The model under review builds one solid part; all positions refer to its coordinate system, in mm. A direction names the side the tool comes from. Round coordinates to 2 decimals unless told otherwise and drop trailing zeros. Order: outer loops, then holes, each group sorted by start corner. A loop starts at its lowest first (then second) coordinate and runs counter-clockwise, first axis right, second up.
1) Clearance check with flat-ended pins moving along their axes: P1, Ø1.8, axis at y = 20, z = 15.5, coming from the -X side; P2, Ø6.5, axis at y = 16, z = -17, coming from the +X side. State where each tip first meets the part, or that it passes through.
2) To check wall thickness, follow L1, parallel to Z at x = -11.5, y = 15.75; L2, parallel to X at y = 9.5, z = 17; L3, parallel to Y at x = -26.5, z = 7. State the ranges of each line that lie inside material, in increasing order.
3) Consider section D-D (y = 22.25). Give the boundary of the cut face in (x, z).
4) Machinability: for faces 4 (the face through (-9, 15, -17)), 5 (the face through (-22, 15, 17)), 6 (the face through (36, 3, 19)), 7 (the face through (-16, 15, -13)), which of the approach directions +Z, -Z, +X, -X, +Y, -Y give a long, thin tool a straight path to every point of the face, cutting with its end or side? Answer none if there is none.
5) Consider section B-B (z = -3.5). Give the boundary of the cut face in (x, y), then the cut area to 3 significant figures.
6) Consider section C-C (x = -4). Give the boundary of the cut face in (y, z).
7) Mouldability with a two-part tool opening along Z and no side actions: class faces 1 (the face through (-38, 2, 0)), 2 (the face through (-16, 15, 13)), 3 (the face through (-7, 4, 20)) as pulls with the +Z half, pulls with the -Z half, needs draft (parallel to the pull), parting line crosses it, or undercut.
8) Consider section A-A (y = 8). Give the boundary of the cut face in (x, z).
from build123d import *

# Parameters (mm, degrees)
SKETCH_1_W          = 76
SKETCH_1_H          = 40
EXTRUDE_1_DEPTH     = 6
SKETCH_2_W          = 13
SKETCH_2_H          = 40
EXTRUDE_2_DEPTH     = 19
SKETCH_3_W          = 13
SKETCH_3_H          = 26
CUT_EXTRUDE_1_DEPTH = 19
FILLET_1_R          = 4
FILLET_2_R          = 1
FILLET_3_R          = 1
FILLET_4_R          = 5
FILLET_5_R          = 1
FILLET_6_R          = 1
FILLET_7_R          = 0.4


with BuildPart() as part:
    # Эскиз1 → Бобышка-Вытянуть1 (new body)
    with BuildSketch(Plane(origin=(0, 0, 0), x_dir=(1, 0, 0), z_dir=(0, 1, 0))):
        Rectangle(SKETCH_1_W, SKETCH_1_H)
    extrude(amount=EXTRUDE_1_DEPTH)

    # Эскиз2 → Бобышка-Вытянуть2 (add)
    with BuildSketch(Plane(origin=(0, 6, 0), x_dir=(1, 0, 0), z_dir=(0, 1, 0))):
        with Locations((-15.5, 0)):
            Rectangle(SKETCH_2_W, SKETCH_2_H)
    extrude(amount=EXTRUDE_2_DEPTH)

    # Эскиз3 → Вырез-Вытянуть1 (cut)
    with BuildSketch(Plane(origin=(0, 25, 0), x_dir=(1, 0, 0), z_dir=(0, 1, 0))):
        with Locations((-15.5, 0)):
            Rectangle(SKETCH_3_W, SKETCH_3_H)
    extrude(amount=-CUT_EXTRUDE_1_DEPTH, mode=Mode.SUBTRACT)

    # Скругление1
    fillet_1_edges = [part.edges().sort_by_distance(p)[0] for p in [
        (-15.5, 25, 20),
        (-15.5, 25, -20),
    ]]
    fillet(fillet_1_edges, radius=FILLET_1_R)

    # Скругление2
    fillet_2_edges = [part.edges().sort_by_distance(p)[0] for p in [
        (-22, 15.5, -13),
        (-9, 15.5, -13),
        (-15.5, 25, -13),
    ]]
    fillet(fillet_2_edges, radius=FILLET_2_R)

    # Скругление3
    fillet_3_edges = [part.edges().sort_by_distance(p)[0] for p in [
        (-22, 15.5, 13),
        (-9, 15.5, 13),
        (-15.5, 25, 13),
    ]]
    fillet(fillet_3_edges, radius=FILLET_3_R)

    # Скругление4
    fillet_4_edges = [part.edges().sort_by_distance(p)[0] for p in [
        (38, 3, 20),
        (-38, 3, 20),
        (-38, 3, -20),
        (38, 3, -20),
    ]]
    fillet(fillet_4_edges, radius=FILLET_4_R)

    # Скругление5
    fillet_5_edges = [part.edges().sort_by_distance(p)[0] for p in [
        (-38, 6, 0),
        (-27.5, 6, 20),
        (-36.535533906, 6, 18.535533906),
        (-36.535533906, 6, -18.535533906),
        (-27.5, 6, -20),
    ]]
    fillet(fillet_5_edges, radius=FILLET_5_R)

    # Скругление6
    fillet_6_edges = [part.edges().sort_by_distance(p)[0] for p in [
        (12, 6, -20),
        (38, 6, 0),
        (36.535533906, 6, -18.535533906),
        (36.535533906, 6, 18.535533906),
        (12, 6, 20),
    ]]
    fillet(fillet_6_edges, radius=FILLET_6_R)

    # Скругление7
    # the kernel refuses this fillet: 0.4 mm, written as the material it adds along each edge
    with BuildSketch(Plane(origin=(-22, 6, -19), x_dir=(-1, 0, 0), z_dir=(0, 0, 1)), Plane(origin=(-9, 6, 19), x_dir=(1, 0, 0), z_dir=(0, 0, -1)), Plane(origin=(-9, 6, -14), x_dir=(1, 0, 0), z_dir=(0, 0, -1)), Plane(origin=(-22, 6, 14), x_dir=(-1, 0, 0), z_dir=(0, 0, 1))) as fillet_7_piece_1:
        with BuildLine():
            CenterArc((FILLET_7_R, -FILLET_7_R), FILLET_7_R, 90, 90)
            Line((0, -FILLET_7_R), (0, 0))
            Line((0, 0), (FILLET_7_R, 0))
        make_face()
    extrude(amount=5)
    with BuildSketch(Plane(origin=(-22, 5, -19), x_dir=(0, 1, 0), z_dir=(0, 0, 1))) as fillet_7_piece_2_section:
        with BuildLine():
            CenterArc((1 + FILLET_7_R, FILLET_7_R), FILLET_7_R, 180, 90)
            Line((1, FILLET_7_R), (1, 0))
            Line((1, 0), (1 + FILLET_7_R, 0))
        make_face()
    fillet_7_piece_2 = revolve(axis=Axis((-22, 5, -19), (-1, 0, 0)), revolution_arc=147.318795695, mode=Mode.PRIVATE)
    fillet_7_piece_2 = split(fillet_7_piece_2, bisect_by=Plane(origin=(-22.06536945, 6.084454663, -20), z_dir=(0, 0, 1)), keep=Keep.TOP, mode=Mode.PRIVATE)
    add(fillet_7_piece_2)
    with BuildSketch(Plane(origin=(-22, 5, 19), x_dir=(0, 1, 0), z_dir=(0, 0, -1))) as fillet_7_piece_3_section:
        with BuildLine():
            CenterArc((1 + FILLET_7_R, -FILLET_7_R), FILLET_7_R, 90, 90)
            Line((1 + FILLET_7_R, 0), (1, 0))
            Line((1, 0), (1, -FILLET_7_R))
        make_face()
    fillet_7_piece_3 = revolve(axis=Axis((-22, 5, 19), (1, 0, 0)), revolution_arc=147.318795695, mode=Mode.PRIVATE)
    fillet_7_piece_3 = split(fillet_7_piece_3, bisect_by=Plane(origin=(-22.10538555, 5.722614098, 20), z_dir=(0, 0, -1)), keep=Keep.TOP, mode=Mode.PRIVATE)
    add(fillet_7_piece_3)
    with BuildSketch(Plane(origin=(-9, 5, -19), x_dir=(0, 1, 0), z_dir=(0, 0, 1))) as fillet_7_piece_4_section:
        with BuildLine():
            CenterArc((1 + FILLET_7_R, -FILLET_7_R), FILLET_7_R, 90, 90)
            Line((1, -FILLET_7_R), (1, 0))
            Line((1, 0), (1 + FILLET_7_R, 0))
        make_face()
    fillet_7_piece_4 = revolve(axis=Axis((-9, 5, -19), (-1, 0, 0)), revolution_arc=147.318795695, mode=Mode.PRIVATE)
    fillet_7_piece_4 = split(fillet_7_piece_4, bisect_by=Plane(origin=(-8.934630555, 6.084454665, -20), z_dir=(0, 0, 1)), keep=Keep.TOP, mode=Mode.PRIVATE)
    add(fillet_7_piece_4)
    with BuildSketch(Plane(origin=(-9, 5, 19), x_dir=(0, 1, 0), z_dir=(0, 0, -1))) as fillet_7_piece_5_section:
        with BuildLine():
            CenterArc((1 + FILLET_7_R, FILLET_7_R), FILLET_7_R, 180, 90)
            Line((1 + FILLET_7_R, 0), (1, 0))
            Line((1, 0), (1, FILLET_7_R))
        make_face()
    fillet_7_piece_5 = revolve(axis=Axis((-9, 5, 19), (1, 0, 0)), revolution_arc=147.318795695, mode=Mode.PRIVATE)
    fillet_7_piece_5 = split(fillet_7_piece_5, bisect_by=Plane(origin=(-8.894614474, 5.72261425, 20), z_dir=(0, 0, -1)), keep=Keep.TOP, mode=Mode.PRIVATE)
    add(fillet_7_piece_5)
    with BuildSketch(Plane(origin=(-21, 6, -13), x_dir=(0, 0, 1), z_dir=(1, 0, 0)), Plane(origin=(-10, 6, 13), x_dir=(0, 0, -1), z_dir=(-1, 0, 0))) as fillet_7_piece_6:
        with BuildLine():
            CenterArc((FILLET_7_R, -FILLET_7_R), FILLET_7_R, 90, 90)
            Line((0, -FILLET_7_R), (0, 0))
            Line((0, 0), (FILLET_7_R, 0))
        make_face()
    extrude(amount=11)
    with BuildSketch(Plane(origin=(-10, 6, -14), x_dir=(1, 0, 0), z_dir=(0, 0, -1))) as fillet_7_piece_7:
        with BuildLine():
            CenterArc((1 + FILLET_7_R, -FILLET_7_R), FILLET_7_R, 90, 90)
            Line((1, -FILLET_7_R), (1, 0))
            Line((1, 0), (1 + FILLET_7_R, 0))
        make_face()
    revolve(axis=Axis((-10, 6, -14), (0, -1, 0)), revolution_arc=90)
    with BuildSketch(Plane(origin=(-21, 6, -14), x_dir=(0, 0, 1), z_dir=(1, 0, 0))) as fillet_7_piece_8:
        with BuildLine():
            CenterArc((1 + FILLET_7_R, -FILLET_7_R), FILLET_7_R, 90, 90)
            Line((1, -FILLET_7_R), (1, 0))
            Line((1, 0), (1 + FILLET_7_R, 0))
        make_face()
    revolve(axis=Axis((-21, 6, -14), (0, -1, 0)), revolution_arc=90)
    with BuildSketch(Plane(origin=(-10, 6, 14), x_dir=(1, 0, 0), z_dir=(0, 0, 1))) as fillet_7_piece_9:
        with BuildLine():
            CenterArc((1 + FILLET_7_R, FILLET_7_R), FILLET_7_R, 180, 90)
            Line((1, FILLET_7_R), (1, 0))
            Line((1, 0), (1 + FILLET_7_R, 0))
        make_face()
    revolve(axis=Axis((-10, 6, 14), (0, 1, 0)), revolution_arc=90)
    with BuildSketch(Plane(origin=(-21, 6, 14), x_dir=(0, 0, -1), z_dir=(1, 0, 0))) as fillet_7_piece_10:
        with BuildLine():
            CenterArc((1 + FILLET_7_R, FILLET_7_R), FILLET_7_R, 180, 90)
            Line((1, FILLET_7_R), (1, 0))
            Line((1, 0), (1 + FILLET_7_R, 0))
        make_face()
    revolve(axis=Axis((-21, 6, 14), (0, 1, 0)), revolution_arc=90)


solid = part.part
Answer below:
1. P1: stops at x = -22
1. P2: stops at x = -9
2. L1: z = -20 to -13, 13 to 20
2. L2: x = -22 to -9
2. L3: y = 0 to 6
3. outline: (-22, -19.8) - (-9, -19.8) - (-9, -14) arc R1 ccw to (-10, -13) - (-21, -13) arc R1 ccw to (-22, -14) - close; (-22, 14) arc R1 ccw to (-21, 13) - (-10, 13) arc R1 ccw to (-9, 14) - (-9, 19.8) - (-22, 19.8) - close
4. face 4: +Z, -Z, +X, +Y
4. face 5: +Z, -Z, -X, +Y
4. face 6: +Z, +X, +Y, -Y
4. face 7: +X, -X, +Y
5. outline: (-38, 0) - (38, 0) - (38, 5) arc R1 ccw to (37, 6) - (-37, 6) arc R1 ccw to (-38, 5) - close
5. area: 456 mm2
6. outline: (0, -20) - (5, -20) arc R1 ccw to (6, -19) - (6, 19) arc R1 ccw to (5, 20) - (0, 20) - close
7. face 1: needs draft
7. face 2: undercut
7. face 3: pulls with the +Z half
8. outline: (-22, -20) - (-9, -20) - (-9, -14) arc R1 ccw to (-10, -13) - (-21, -13) arc R1 ccw to (-22, -14) - close; (-22, 14) arc R1 ccw to (-21, 13) - (-10, 13) arc R1 ccw to (-9, 14) - (-9, 20) - (-22, 20) - close
